Input: part model. Units: mm. Frame: model coordinates. Face numbers are marked on the shaded views. A direction names the side the tool comes from. Give positions to 0.01 mm unless a question says otherwise; leave off trailing zeros. Loops run counter-clockwise (first coordinate to the right, second up) from the corner with the lowest first, then second, coordinate; pieces in that order, holes last. Notation, with made-up numbers: M 82,54 L 110,54 A20 cw 110,67 Z; hole C -18.5,1 d6. An arc over 180 degrees is marked long. Answer as a JSON object with one key per item and string values. Group by question number.
1) First-contact query: P1, Ø5, axis at y = -48.5, z = 6, coming from the -X side; P2, Ø12, axis at x = -51.5, y = -35.5, coming from the +Z side; P3, Ø4, axis at x = -35, z = 19.5, coming from the -Y side. Flat tips, straight axial feed; report the tip coordinate or a pass-through.
2) Draft query along Y for the marked faces 1, 2, 3 and 4. Return one class per face: +Y half, -Y half, draft (parallel to the pull), parting line (faces both ways), or undercut.
3) Access query for the marked faces 5, 6 and 7. Directions: +Z, -Z, +X, -X, +Y, -Y. A direction counts if a zero-diameter tool reaches every point of the face in a straight line with its end or side. Return the directions, or none.
4) Section query A-A on z = -15.5. Return loops of the section in (x, y), plus the area to 3 significant figures.
5) Section query C-C on z = 6.5. Return loops of the section in (x, y).
6) Section query B-B on y = -25. Return loops of the section in (x, z), plus the area to 3 significant figures.
7) Ray query, L1, parallel to Y at x = -62, z = 21.5; L2, parallel to X at y = 6.5, z = 19.5; L3, parallel to X at y = -17, z = 25. Return the intervals inside material, ascending.
8) Section query D-D on x = 0. Return loops of the section in (y, z), plus the area to 3 significant figures.
from build123d import *

# Parameters (mm, degrees)
F1_DEPTH = 70
F2_W     = 30
F2_H     = 30
F3_DEPTH = 60
F4_R     = 15
F5_DEPTH = 72.5
F6_R     = 5
F7_DEPTH = 37.8
F8_R     = 5
F9_DEPTH = 25


# Not quite as in the source:
# - a pattern or mirror of a feature is missing from the dataset's text; its kind, count and spacing are read off the source's solid


with BuildPart() as f1:
    # F0 (on Right) → F1 (new body, symmetric)
    with BuildSketch(Plane.YZ):
        with BuildLine():
            Line((10, 30), (0, 30))
            Line((0, 30), (0, 0))
            Line((0, 0), (-60, 0))
            Line((-60, 0), (-60, -30))
            Line((-60, -30), (-46.7469906007, -30))
            ThreePointArc((-46.7469906007, -30), (-25, -8.2530093993), (-3.2530093993, -30))
            Line((-3.2530093993, -30), (10, -30))
            Line((10, -30), (10, 30))
        make_face()
    extrude(amount=F1_DEPTH, both=True)

    # F2 (on face) → F3 (join, through all)
    with BuildSketch(Plane.XZ):
        with Locations((15, 15)):
            Rectangle(F2_W, F2_H)
    f3 = extrude(amount=F3_DEPTH)

    # F3_copies: F3 across plane
    add(f3.mirror(Plane(origin=(0, 0, 0), x_dir=(0, 0, -1), z_dir=(-1, 0, 0))))

    # F4 (on face) → F5 (cut)
    with BuildSketch(Plane.XZ.offset(60)):
        with Locations((0, 30)):
            Circle(F4_R)
    extrude(amount=-F5_DEPTH, mode=Mode.SUBTRACT)

    # F6 (on face) → F7 (cut)
    with BuildSketch(Plane.XZ):
        with Locations((48.3254604042, 16.4307225496)):
            Circle(F6_R)
    extrude(amount=-F7_DEPTH, mode=Mode.SUBTRACT)

    # F8 (on face) → F9 (cut)
    with BuildSketch(Plane.XZ):
        with Locations((-53.8972392678, 16.9797260314)):
            Circle(F8_R)
    extrude(amount=-F9_DEPTH, mode=Mode.SUBTRACT)


solid = f1.part
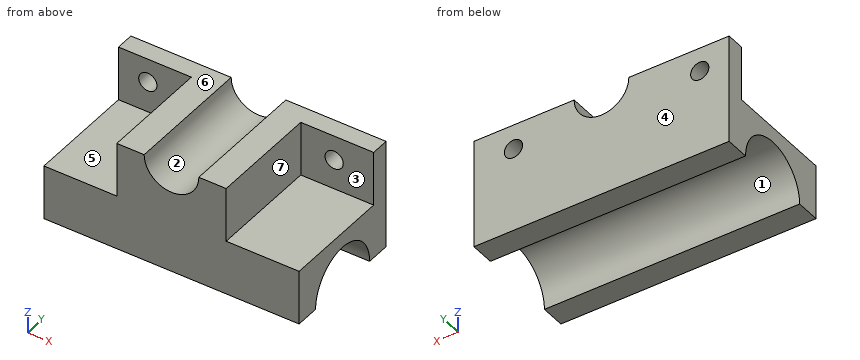
Output:
{
 "1": {"P1": "stops at x = -30", "P2": "stops at z = 0", "P3": "stops at y = 0"},
 "2": {"face 1": "undercut", "face 2": "draft", "face 3": "-Y half", "face 4": "+Y half"},
 "3": {"face 5": "+Z, -X, -Y", "face 6": "+Z, +X, -X, +Y, -Y", "face 7": "+Z, +X, -Y"},
 "4": {"outline": "M -70,-60 L 70,-60 L 70,-41.21 L -70,-41.21 Z; M -70,-8.79 L 70,-8.79 L 70,10 L -70,10 Z", "area": "5,260 mm^2"},
 "5": {"outline": "M -70,0 L -30,0 L -30,-60 L 30,-60 L 30,0 L 70,0 L 70,10 L -70,10 Z"},
 "6": {"outline": "M -70,-8.25 L 70,-8.25 L 70,0 L 30,0 L 30,30 L 15,30 A15 cw -15,30 L -30,30 L -30,0 L -70,0 Z", "area": "2,600 mm^2"},
 "7": {"L1": "y = 0 to 10", "L2": "x = -70 to -58.22, -49.58 to -10.71, 10.71 to 44.38, 52.27 to 70", "L3": "x = -30 to -14.14, 14.14 to 30"},
 "8": {"outline": "M -60,-30 L -46.75,-30 A21.75 cw -3.25,-30 L 10,-30 L 10,15 L -60,15 Z", "area": "2,410 mm^2"}
}
